from build123d import *

# Parameters (mm, degrees)
F0_W     = 152.4
F0_H     = 152.4
F1_DEPTH = 1162.05
F2_T     = -3.175
F3_R     = 25.40254
F4_DEPTH = 3.176
F5_R     = 12.7
F6_DEPTH = 1162.051


with BuildPart() as f1:
    # F0 (on Front) → F1 (new body)
    with BuildSketch(Plane.XZ):
        with Locations((-76.2, 76.2)):
            Rectangle(F0_W, F0_H)
    extrude(amount=F1_DEPTH)

    # F2
    f2_openings = [f1.faces().sort_by_distance(p)[0] for p in [
        (-76.2, -581.025, 152.4),
    ]]
    offset(amount=F2_T, openings=f2_openings)

    # F3 (on face) → F4 (cut, through all)
    with BuildSketch(Plane.XY.offset(3.175)):
        with Locations((-74.6125, -579.4375)):
            Circle(F3_R)
    extrude(amount=-F4_DEPTH, mode=Mode.SUBTRACT)

    # F5 (on face) → F6 (cut, through all)
    with BuildSketch(Plane.XZ.offset(1162.05)):
        with Locations((-44.45, 101.6)):
            Circle(F5_R)
    extrude(amount=-F6_DEPTH, mode=Mode.SUBTRACT)


solid = f1.part
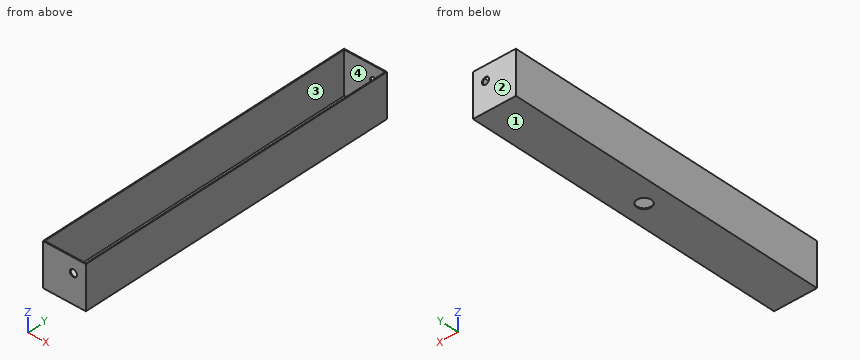
Source: CAD feature listing. Evaluate the final solid. Frame: model axes, mm. Face numbers are marked on the shaded views. Give positions to 0.01 mm unless a question says otherwise; leave off trailing zeros. Order: outer loops, then holes, each group sorted by start corner. A loop starts at its lowest first (then second) coordinate and runs counter-clockwise, first axis right, second up. Notation, with made-up numbers: (30, -10.75) -> (53, -10.75) arc R26 cw to (53, 3.25) -> close; hole circle Ø4 at (39.25, -37). An arc over 180 degrees is marked (long way). Use a Markdown table: item, result.
1) Section query C-C, the plane y = -104. Return the cut outline in (x, z) (3 decimals), then the cut area to 3 significant figures.
Answer list:
| item | result |
|---|---|
| outline | (-152.4, 0) -> (0, 0) -> (0, 152.4) -> (-3.175, 152.4) -> (-3.175, 3.175) -> (-149.225, 3.175) -> (-149.225, 152.4) -> (-152.4, 152.4) -> close |
| area | 1,430 mm² |
2) Section query B-B, the plane z = 46. Return the cut outline in (x, y) (3 decimals), then the cut area to 3 significant figures.
Answer list:
| item | result |
|---|---|
| outline | (-152.4, -1162.05) -> (0, -1162.05) -> (0, 0) -> (-152.4, 0) -> close; hole (-149.225, -1158.875) -> (-3.175, -1158.875) -> (-3.175, -3.175) -> (-149.225, -3.175) -> close |
| area | 8,310 mm² |
3) Ray query, line 1 along Y through (x, z) = (-100.5, 50) (3 decimals); line 2 along X through (y, z) = (-617, 23.5) (3 decimals); line 3 along Z through (x, y) = (-44.45, -1161.1). Return the intervals inside material, ascending. Write a range as [from, to].
Answer list:
| item | result |
|---|---|
| line 1 | [-1162.05, -1158.875], [-3.175, 0] |
| line 2 | [-152.4, -149.225], [-3.175, 0] |
| line 3 | [0, 88.9], [114.3, 152.4] |
4) Contact query for flat-ended pins moving along their axis: P1, Ø12, axis at x = -117, y = -885, coming from the +Z side (3 decimals); P2, Ø15, axis at x = -44.45, z = 101.6, coming from the -Y side; P3, Ø12, axis at x = -73, z = 53.5, coming from the +Y side. Output: stop coordinate, or through.
Answer list:
| item | result |
|---|---|
| P1 | z = 3.175 |
| P2 | through |
| P3 | y = 0 |
5) Mould query, pull axis Y, two halves, no side actions, for the marked faces 1, 2, 3 and 4. Classes: +Y half, -Y half, draft (parallel to the pull), parting line (faces both ways), or undercut.
Answer list:
| item | result |
|---|---|
| face 1 | draft |
| face 2 | +Y half |
| face 3 | undercut |
| face 4 | undercut |
6) Section query A-A, the plane z = 101.6. Return the cut outline in (x, y) (3 decimals).
Answer list:
| item | result |
|---|---|
| outline | (-152.4, -1162.05) -> (-57.15, -1162.05) -> (-57.15, -1158.875) -> (-149.225, -1158.875) -> (-149.225, -3.175) -> (-57.15, -3.175) -> (-57.15, 0) -> (-152.4, 0) -> close; (-31.75, -1162.05) -> (0, -1162.05) -> (0, 0) -> (-31.75, 0) -> (-31.75, -3.175) -> (-3.175, -3.175) -> (-3.175, -1158.875) -> (-31.75, -1158.875) -> close |
